Part model, mm, in its own coordinate system. A direction names the side the tool comes from. Round coordinates to 2 decimals unless told otherwise and drop trailing zeros. Loops run counter-clockwise (first coordinate to the right, second up) from the corner with the lowest first, then second, coordinate; pieces in that order, holes last.
(1) Mould opens along X. For faces 4 (the face through (0, 0, -4.762)), 5 (the face through (1.588, 0, -8)), 6 (the face through (5.13, -2.13, -4.7)), 7 (the face through (0, -4, 0)) say: +X half, -X half, draft (parallel to the pull), parting line (faces both ways), or undercut.
(2) Probe probe 1 along Y at (x, z) = (0, -2.45); probe 2 along X at (y, z) = (-1, -0.75); probe 3 along Z at (x, y) = (1.75, -2.5) (1 decimal). List the from-to ranges inside material, lowest first.
(3) Tool access for faces 1 (the face through (3.05, -1.26, -2.35)), 2 (the face through (0, 0, -6.35)), 3 (the face through (-3, 0, -9.525)): list every direction of +Z, -Z, +X, -X, +Y, -Y with a clear straight run to the whole face (end or side of a thin tool).
(4) Flat gauge pins, fed straight in: pin 1 (1 mm diameter, centred on y = -1, z = -1.5, fed in from -X); pin 2 (1.5 mm diameter, centred on x = 1, y = 0, fed in from +Z); pin 3 (1 mm diameter, centred on x = -0.5, y = -0.5, fed in from -Z). Where does each tip first touch, or does it go through?
(5) Cut at C-C on x = 0. List the corners of the cut face in (y, z), then the cut area to 3 significant figures.
(6) Cut at A-A on z = -6.5. List the corners of the cut face in (x, y).
(7) Cut at D-D on z = -4.5. List the corners of the cut face in (x, y).
from build123d import *

# Parameters (mm, degrees)
F0_R     = 5.55625
F1_DEPTH = 9.525
F2_W     = 3.175
F2_H     = 11.1125
F3_DEPTH = 3.175
F4_R     = 3.302
F5_DEPTH = 4.7625


with BuildPart() as f1:
    # F0 (on Top) → F1 (new body)
    with BuildSketch(Plane.XY):
        Circle(F0_R)
    extrude(amount=-F1_DEPTH)

    # F2 (on face) → F3 (cut)
    with BuildSketch(Plane(origin=(0, 0, -9.525), x_dir=(1, 0, 0), z_dir=(0, 0, -1))):
        Rectangle(F2_W, F2_H)
    extrude(amount=-F3_DEPTH, mode=Mode.SUBTRACT)

    # F4 (on face) → F5 (cut)
    with BuildSketch(Plane.XY):
        Circle(F4_R)
    extrude(amount=-F5_DEPTH, mode=Mode.SUBTRACT)


solid = f1.part
Final values:
1. face 4: undercut
1. face 5: undercut
1. face 6: parting line
1. face 7: draft
2. probe 1: y = -5.56 to -3.3, 3.3 to 5.56
2. probe 2: x = -5.47 to -3.15, 3.15 to 5.47
2. probe 3: z = -9.5 to -4.8
3. face 1: +Z
3. face 2: -Z, +Y, -Y
3. face 3: -Z, +X, -X, +Y, -Y
4. pin 1: stops at x = -5.53
4. pin 2: stops at z = -4.76
4. pin 3: stops at z = -6.35
5. outline: (-5.56, -6.35) - (5.56, -6.35) - (5.56, 0) - (3.3, 0) - (3.3, -4.76) - (-3.3, -4.76) - (-3.3, 0) - (-5.56, 0) - close
5. area: 39.1 mm2
6. outline: (-1.59, -5.32) - (-1.59, 5.32) arc R5.56 ccw to start; (1.59, -5.32) arc R5.56 ccw to (1.59, 5.32) - close
7. outline: circle Ø11.11 at (0, 0); hole circle Ø6.6 at (0, 0)
